```python
from build123d import *

# Parameters (mm, degrees)
F1_DEPTH = 14.224
F2_DEPTH = 7.874
F3_DEPTH = 12.7
F0_W     = 6.35
F0_H     = 28.575
F4_DEPTH = 7.874
F5_DEPTH = 3.048


with BuildPart() as f1:
    # F0 (on Top) → F1 (new body, symmetric)
    with BuildSketch(Plane.XY):
        Polygon((-30.353, 15.875), (-36.703, 15.875), (-36.703, -15.875), (-30.353, -15.875), (36.703, -15.875), (36.703, 15.875), align=None)
    extrude(amount=F1_DEPTH, both=True)

    # F0 (on Top) → F2 (join, symmetric)
    with BuildSketch(Plane.XY):
        Polygon((-30.353, 44.45), (-30.353, 15.875), (36.703, 15.875), (39.37, 15.875), (50.419, 26.924), (32.893, 26.924), (32.893, 44.45), align=None)
        with BuildLine():
            ThreePointArc((-6.477, 24.638), (-12.065, 30.226), (-6.477, 35.814))
            Line((-6.477, 35.814), (17.399, 35.814))
            ThreePointArc((17.399, 35.814), (22.987, 30.226), (17.399, 24.638))
            Line((17.399, 24.638), (-6.477, 24.638))
        make_face(mode=Mode.SUBTRACT)
        Polygon((36.703, -15.875), (-30.353, -15.875), (-30.353, -44.45), (32.893, -44.45), (32.893, -26.924), (50.419, -26.924), (39.37, -15.875), align=None)
        with BuildLine():
            Line((-6.477, -24.638), (17.399, -24.638))
            ThreePointArc((17.399, -24.638), (22.987, -30.226), (17.399, -35.814))
            Line((17.399, -35.814), (-6.477, -35.814))
            ThreePointArc((-6.477, -35.814), (-12.065, -30.226), (-6.477, -24.638))
        make_face(mode=Mode.SUBTRACT)
    extrude(amount=F2_DEPTH, both=True)

    # F0 (on Top) → F3 (join, symmetric)
    with BuildSketch(Plane.XY):
        Polygon((67.945, 44.45), (32.893, 44.45), (32.893, 26.924), (50.419, 26.924), align=None)
        Polygon((32.893, -26.924), (32.893, -44.45), (67.945, -44.45), (50.419, -26.924), align=None)
    extrude(amount=F3_DEPTH, both=True)

    # F0 (on Top) → F4 (join)
    with BuildSketch(Plane.XY):
        with Locations((-33.528, 30.1625)):
            Rectangle(F0_W, F0_H)
        with Locations((-33.528, -30.1625)):
            Rectangle(F0_W, F0_H)
    extrude(amount=-F4_DEPTH)

    # F0 (on Top) → F5 (join)
    with BuildSketch(Plane.XY):
        with Locations((-33.528, 30.1625)):
            Rectangle(F0_W, F0_H)
        with Locations((-33.528, -30.1625)):
            Rectangle(F0_W, F0_H)
    extrude(amount=F5_DEPTH)


solid = f1.part
```
Geometry check sheet. Reference: the model listing, model coordinates, mm. A direction names the side the tool comes from. Round coordinates to 2 decimals unless told otherwise and drop trailing zeros. Loops run counter-clockwise (first coordinate to the right, second up) from the corner with the lowest first, then second, coordinate; pieces in that order, holes last. Notation, with made-up numbers: (-14, 54.5) -> (36, 54.5) arc R35 cw to (36, 87.5) -> close; hole circle Ø10 at (59, 4.5). An arc over 180 degrees is marked (long way). Use a Markdown table: item, result.
(1) Set-up check for faces 1 (the flat face through (38, -15.875, 0)), 2 (the flat face through (42, 26.924, 10)), 3 (the flat face through (6, 24.638, 0)), 4 (the flat face through (46, -36, -12.7)): record each of +Z, -Z, +X, -X, +Y, -Y from which the full face is reachable in a straight line by a thin tool's end or side.
Calculated:
| item | result |
|---|---|
| face 1 | +Z, -Z, +X |
| face 2 | +Z, +X, -X |
| face 3 | +Z, -Z |
| face 4 | -Z, +X, -X, -Y |
(2) Sectioned sample at A-A (x = -2.5). Enter the section's corners in (y, z) (3 decimals).
Calculated:
| item | result |
|---|---|
| outline | (-44.45, -7.874) -> (-35.814, -7.874) -> (-35.814, 7.874) -> (-44.45, 7.874) -> close; (-24.638, -7.874) -> (-15.875, -7.874) -> (-15.875, -14.224) -> (15.875, -14.224) -> (15.875, -7.874) -> (24.638, -7.874) -> (24.638, 7.874) -> (15.875, 7.874) -> (15.875, 14.224) -> (-15.875, 14.224) -> (-15.875, 7.874) -> (-24.638, 7.874) -> close; (35.814, -7.874) -> (44.45, -7.874) -> (44.45, 7.874) -> (35.814, 7.874) -> close |
(3) Go/stop test with flat-tipped pins: P1, Ø1, axis at x = -10.5, y = -19.5, coming from the -Z side; P2, Ø3, axis at x = -8.5, z = -10.5, coming from the +Y side (3 decimals); P3, Ø19.5, axis at x = 56, y = 32.5, coming from the -Z side; P4, Ø10, axis at x = 29, y = -18.5, coming from the -Z side. Record where each tip stops, or that it passes through.
Calculated:
| item | result |
|---|---|
| P1 | z = -7.87 |
| P2 | y = 15.875 |
| P3 | z = -12.7 |
| P4 | z = -14.22 |
(4) Sectioned sample at B-B (z = -10.75). Enter the section's corners in (x, y) (3 decimals).
Calculated:
| item | result |
|---|---|
| outline | (-36.703, -15.875) -> (36.703, -15.875) -> (36.703, 15.875) -> (-36.703, 15.875) -> close; (32.893, -44.45) -> (67.945, -44.45) -> (50.419, -26.924) -> (32.893, -26.924) -> close; (32.893, 26.924) -> (50.419, 26.924) -> (67.945, 44.45) -> (32.893, 44.45) -> close |
(5) Sectioned sample at D-D (z = 4.5). Enter the section's corners in (x, y) (3 decimals), then the cut area to 3 significant figures.
Calculated:
| item | result |
|---|---|
| outline | (-36.703, -15.875) -> (-30.353, -15.875) -> (-30.353, -44.45) -> (67.945, -44.45) -> (39.37, -15.875) -> (36.703, -15.875) -> (36.703, 15.875) -> (39.37, 15.875) -> (67.945, 44.45) -> (-30.353, 44.45) -> (-30.353, 15.875) -> (-36.703, 15.875) -> close; hole (-6.477, -35.814) -> (17.399, -35.814) arc R5.588 ccw to (17.399, -24.638) -> (-6.477, -24.638) arc R5.588 ccw to start; hole (-6.477, 24.638) -> (17.399, 24.638) arc R5.588 ccw to (17.399, 35.814) -> (-6.477, 35.814) arc R5.588 ccw to start |
| area | 6,400 mm² |
(6) Mould release check, pull along Y, two halves, no side actions. Record for faces 5 (the flat face through (42, -26.924, 10)), 6 (the flat face through (32.893, -36, -10)): released by +Y, released by -Y, zero draft, split by the parting line, or undercut.
Calculated:
| item | result |
|---|---|
| face 5 | undercut |
| face 6 | zero draft |
(7) Sectioned sample at C-C (x = 61.5). Enter the section's corners in (y, z) (3 decimals).
Calculated:
| item | result |
|---|---|
| outline | (-44.45, -12.7) -> (-38.005, -12.7) -> (-38.005, 12.7) -> (-44.45, 12.7) -> close; (38.005, -12.7) -> (44.45, -12.7) -> (44.45, 12.7) -> (38.005, 12.7) -> close |
(8) Scan lines: probe 1 along Y at (x, z) = (0.5, 1.5); probe 2 along Y at (x, z) = (41, -11.5); probe 3 along X at (y, z) = (9.5, 4.75). Record each from-to range of solid material in increasing order.
Calculated:
| item | result |
|---|---|
| probe 1 | -44.45 to -35.81, -24.64 to 24.64, 35.81 to 44.45 |
| probe 2 | -44.45 to -26.92, 26.92 to 44.45 |
| probe 3 | -36.7 to 36.7 |
